Verification items for this drawing (mm, ordinates from the low corner). A direction names the side the tool comes from. Give positions to 0.01 mm unless a question says otherwise; leave off trailing zeros. Write each loop counter-clockwise with the first axis right and the second up, starting at its lowest first coordinate (ties: lowest second). Pieces come first, ordered by that corner, then holes. Notation, with made-up numbers: (80.5, -38.75) -> (90.5, -38.75) arc R23 ccw to (90.5, -28.75) -> close; hole circle Ø8 at (54, -25.5). An arc over 180 degrees is marked (long way). Use one line per item in the form item = value. Start each with the question number.
(1) Section check D-D, the plane z = 11. Record the cut outline in (x, y).
(2) Section check B-B, the plane y = 55. Record the cut outline in (x, z), plus the area to 3 significant figures.
(3) Section check C-C, the plane y = 12.5. Record the cut outline in (x, z).
(4) Release check for a two-part mould opening along X. For the marked faces 3, 4 and 5 record: pulls with the +X half, pulls with the -X half, needs draft (parallel to the pull), parting line crosses it, or undercut.
(5) Set-up check for the marked faces 1 and 2: record each of +Z, -Z, +X, -X, +Y, -Y from which the full face is reachable in a straight line by a thin tool's end or side.
(6) Scan lines: L1, parallel to Y at x = 342.6, z = 27.5; L2, parallel to X at y = 33.5, z = 26; L3, parallel to Y at x = 107, z = 49. Record each from-to range of solid material in increasing order.
(7) Section check A-A, the plane z = 27.5. Record the cut outline in (x, y).
(8) Depth check by flat-ended pin: pin 1 Ø6 at (x, z) = (215, 38.5) entering from +Y. Enter the tip coordinate at first touch or a pass-through.
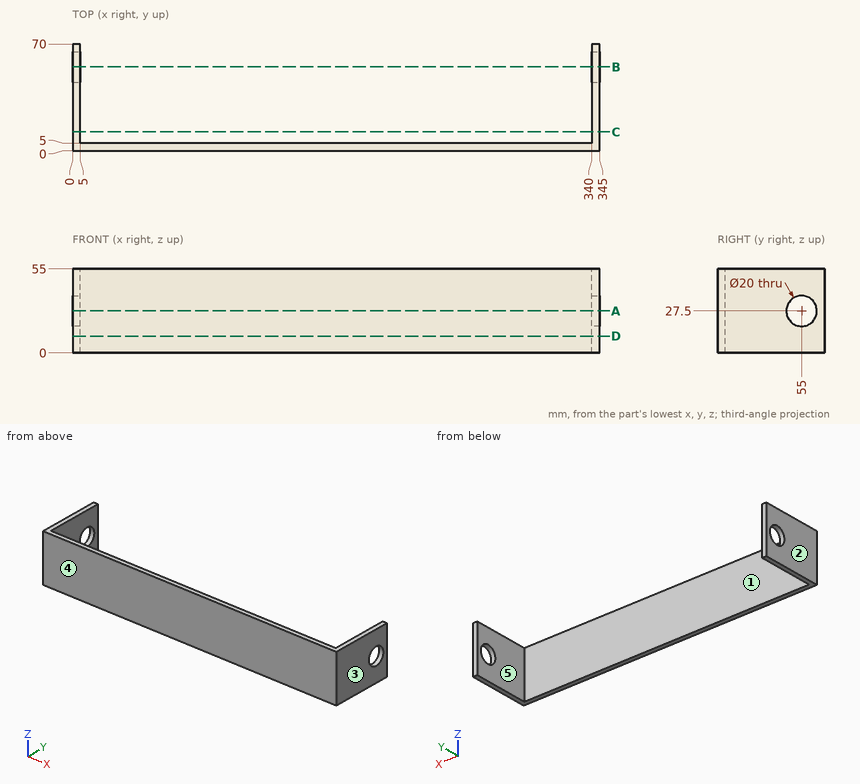
Completed:
q1.outline = (0, 0) -> (345, 0) -> (345, 70) -> (340, 70) -> (340, 5) -> (5, 5) -> (5, 70) -> (0, 70) -> close
q2.outline = (0, 0) -> (5, 0) -> (5, 17.5) -> (0, 17.5) -> close; (0, 37.5) -> (5, 37.5) -> (5, 55) -> (0, 55) -> close; (340, 0) -> (345, 0) -> (345, 17.5) -> (340, 17.5) -> close; (340, 37.5) -> (345, 37.5) -> (345, 55) -> (340, 55) -> close
q2.area = 350 mm²
q3.outline = (0, 0) -> (5, 0) -> (5, 55) -> (0, 55) -> close; (340, 0) -> (345, 0) -> (345, 55) -> (340, 55) -> close
q4.face_3 = pulls with the +X half
q4.face_4 = needs draft
q4.face_5 = undercut
q5.face_1 = +Z, -Z, +Y
q5.face_2 = +Z, -Z, -X, +Y, -Y
q6.L1 = 0 to 45, 65 to 70
q6.L2 = 0 to 5, 340 to 345
q6.L3 = 0 to 5
q7.outline = (0, 0) -> (345, 0) -> (345, 45) -> (340, 45) -> (340, 5) -> (5, 5) -> (5, 45) -> (0, 45) -> close; (0, 65) -> (5, 65) -> (5, 70) -> (0, 70) -> close; (340, 65) -> (345, 65) -> (345, 70) -> (340, 70) -> close
q8.pin_1 = 5
